from build123d import *

# Parameters (mm, degrees)
MODEL_R                 = 4.5
MODEL_W                 = 10
MODEL_H                 = 3
SALIENTE_EXTRUIR1_DEPTH = 3


with BuildPart() as part:
    # Model → Saliente-Extruir1 (new body)
    with BuildSketch(Plane.XY):
        with BuildLine():
            Line((17.831945339, 53.688342713), (41.944056128, 53.688342713))
            Line((41.944056128, 53.688342713), (62.686495879, 53.688342713))
            Line((62.686495879, 53.688342713), (72.203528383, 53.688342713))
            ThreePointArc((72.203528383, 53.688342713), (75.739062289, 52.223876619), (77.203528383, 48.688342713))
            Line((77.203528383, 48.688342713), (77.200462039, 40.688342713))
            Line((77.200462039, 40.688342713), (77.203528383, 29.009907229))
            Line((77.203528383, 29.009907229), (77.203528383, 19.550667198))
            Line((77.203528383, 19.550667198), (77.203528383, 10.10455356))
            Line((77.203528383, 10.10455356), (65.403528383, 10.10455356))
            Line((65.403528383, 10.10455356), (65.403528383, -13.09544644))
            Line((65.403528383, -13.09544644), (77.203528383, -13.09544644))
            Line((77.203528383, -13.09544644), (77.203528383, -33.19043659))
            Line((77.203528383, -33.19043659), (77.203528383, -38.49544644))
            ThreePointArc((77.203528383, -38.49544644), (75.739062152, -42.030980095), (72.203528383, -43.495446053))
            Line((72.203528383, -43.495446053), (0.206594728, -43.495446053))
            ThreePointArc((0.206594728, -43.495446053), (-3.328939178, -42.030979958), (-4.793405272, -38.495446053))
            Line((-4.793405272, -38.495446053), (-4.793405272, -13.09544644))
            Line((-4.793405272, -13.09544644), (7.006594728, -13.09544644))
            Line((7.006594728, -13.09544644), (7.006594728, 10.10455356))
            Line((7.006594728, 10.10455356), (-4.793405272, 10.10455356))
            Line((-4.793405272, 10.10455356), (-4.793405272, 40.688342713))
            Line((-4.793405272, 40.688342713), (-4.793405272, 48.688342713))
            ThreePointArc((-4.793405272, 48.688342713), (-3.328939178, 52.223876619), (0.206594728, 53.688342713))
            Line((0.206594728, 53.688342713), (6.681518597, 53.688342713))
            Line((6.681518597, 53.688342713), (17.831945339, 53.688342713))
        make_face()
        with Locations((69.303528383, -35.49544644)):
            Circle(MODEL_R, mode=Mode.SUBTRACT)
        with Locations((3.103528383, -35.49544644)):
            Circle(MODEL_R, mode=Mode.SUBTRACT)
        with Locations((22.203528383, 47.188342713)):
            Rectangle(MODEL_W, MODEL_H, mode=Mode.SUBTRACT)
        with Locations((50.203528383, 47.188342713)):
            Rectangle(MODEL_W, MODEL_H, mode=Mode.SUBTRACT)
    extrude(amount=SALIENTE_EXTRUIR1_DEPTH)


solid = part.part
Source: CAD feature listing. Evaluate the final solid. Frame: model axes, mm. A direction names the side the tool comes from. Round coordinates to 2 decimals unless told otherwise and drop trailing zeros. Loops run counter-clockwise (first coordinate to the right, second up) from the corner with the lowest first, then second, coordinate; pieces in that order, holes last. Notation, with made-up numbers: (-2, 46.25) - (48, 46.25) arc R9 ccw to (48, 50.25) - close; hole circle Ø6 at (16.25, -21). An arc over 180 degrees is marked (long way). Write item = value, one per line. Start each with the question number.
Item 1: Section query B-B on y = -10.5. Output: boundary loops of the cut face in (x, z), plus the area to 3 significant figures.
Item 2: First-contact query: pin 1 Ø0.9 at (y, z) = (1.5, 2) entering from +X. Flat tip, straight axial feed; report the tip coordinate or a pass-through.
Item 3: Reachability of faces 1 (the face through (45.204, 47, 1)), 2 (the face through (36, 53.688, 1)), 3 (the face through (65.404, -1, 1)) from +Z, -Z, +X, -X, +Y, -Y: full face, straight path, thin tool, end or side. Return the list, or none.
Item 4: Mould query, pull axis X, two halves, no side actions, for faces 4 (the face through (55.204, 47, 1)), 5 (the face through (77.204, -26, 1)), 6 (the face through (37, 6, 0)). Classes: released by +X, released by -X, zero draft, split by the parting line, or undercut.
Item 5: Material intervals for line 1 (Y direction, x = 69.5, z = 1.6); line 2 (X direction, y = 46, z = 2.65); line 3 (Y direction, x = 2, z = 2), sorted ascending.
Item 6: Section query A-A on x = 69. Output: boundary loops of the cut face in (y, z).
Item 7: Section query C-C on z = 1.4. Output: boundary loops of the cut face in (x, y), plus the area to 3 significant figures.
Results list:
q1.outline = (7.01, 0) - (65.4, 0) - (65.4, 3) - (7.01, 3) - close
q1.area = 175 mm²
q2.pin_1 = 65.4
q3.face_1 = +Z, -Z
q3.face_2 = +Z, -Z, +X, -X, +Y
q3.face_3 = +Z, -Z, +X
q4.face_4 = undercut
q4.face_5 = released by +X
q4.face_6 = zero draft
q5.line_1 = -43.5 to -39.99, -31 to -13.1, 10.1 to 53.69
q5.line_2 = -4.79 to 17.2, 27.2 to 45.2, 55.2 to 77.2
q5.line_3 = -43.5 to -39.86, -31.13 to -13.1, 10.1 to 53.69
q6.outline = (-43.5, 0) - (-39.99, 0) - (-39.99, 3) - (-43.5, 3) - close; (-31.01, 0) - (-13.1, 0) - (-13.1, 3) - (-31.01, 3) - close; (10.1, 0) - (53.69, 0) - (53.69, 3) - (10.1, 3) - close
q7.outline = (-4.79, -38.5) arc R5 ccw to (0.21, -43.5) - (72.2, -43.5) arc R5 ccw to (77.2, -38.5) - (77.2, -13.1) - (65.4, -13.1) - (65.4, 10.1) - (77.2, 10.1) - (77.2, 29.01) - (77.2, 40.69) - (77.2, 48.69) arc R5 ccw to (72.2, 53.69) - (0.21, 53.69) arc R5 ccw to (-4.79, 48.69) - (-4.79, 10.1) - (7.01, 10.1) - (7.01, -13.1) - (-4.79, -13.1) - close; hole circle Ø9 at (3.1, -35.5); hole (17.2, 45.69) - (27.2, 45.69) - (27.2, 48.69) - (17.2, 48.69) - close; hole (45.2, 45.69) - (55.2, 45.69) - (55.2, 48.69) - (45.2, 48.69) - close; hole circle Ø9 at (69.3, -35.5)
q7.area = 7,210 mm²
